Geometry: see drawing. Coordinates: mm, zero at the bounding-box minimum. A direction names the side the tool comes from. Coordinates: 2 decimals unless noted, no trailing zeros. Write each loop counter-clockwise with the first axis right and the second up, starting at its lowest first coordinate (ties: lowest second). Pieces come first, ordered by that corner, then holes. Notation, with made-up numbers: (47.5, 40.25) -> (106.5, 40.25) arc R21 ccw to (106.5, 72.25) -> close; hole circle Ø11 at (78, 37.5). An arc over 180 degrees is marked (long way). Use one line per item in the form item = value. Start each with the question number.
(1) First-contact query: pin 1 (12 mm diameter, centred on x = 38, z = 31.5, fed in from -Y); pin 2 (12.5 mm diameter, centred on y = 16.5, z = 35, fed in from +X). Flat tips, straight axial feed; report the tip coordinate or a pass-through.
(2) Ray query, line 1 along X through (y, z) = (24, 38.5); line 2 along Z through (x, y) = (36, 25); line 3 along Y through (x, z) = (43.5, 27). Return the intervals inside material, ascending.
(3) Set-up query: the marked faces 1 and 2. Return all of +Z, -Z, +X, -X, +Y, -Y with unobstructed straight access to the full face (end or side cutting, diameter ignored); none if empty.
(4) Cut plane A-A on y = 17.5. Return the cut outline in (x, z), plus the area to 3 significant figures.
(5) Cut plane B-B on x = 47. Return the cut outline in (y, z), plus the area to 3 significant figures.
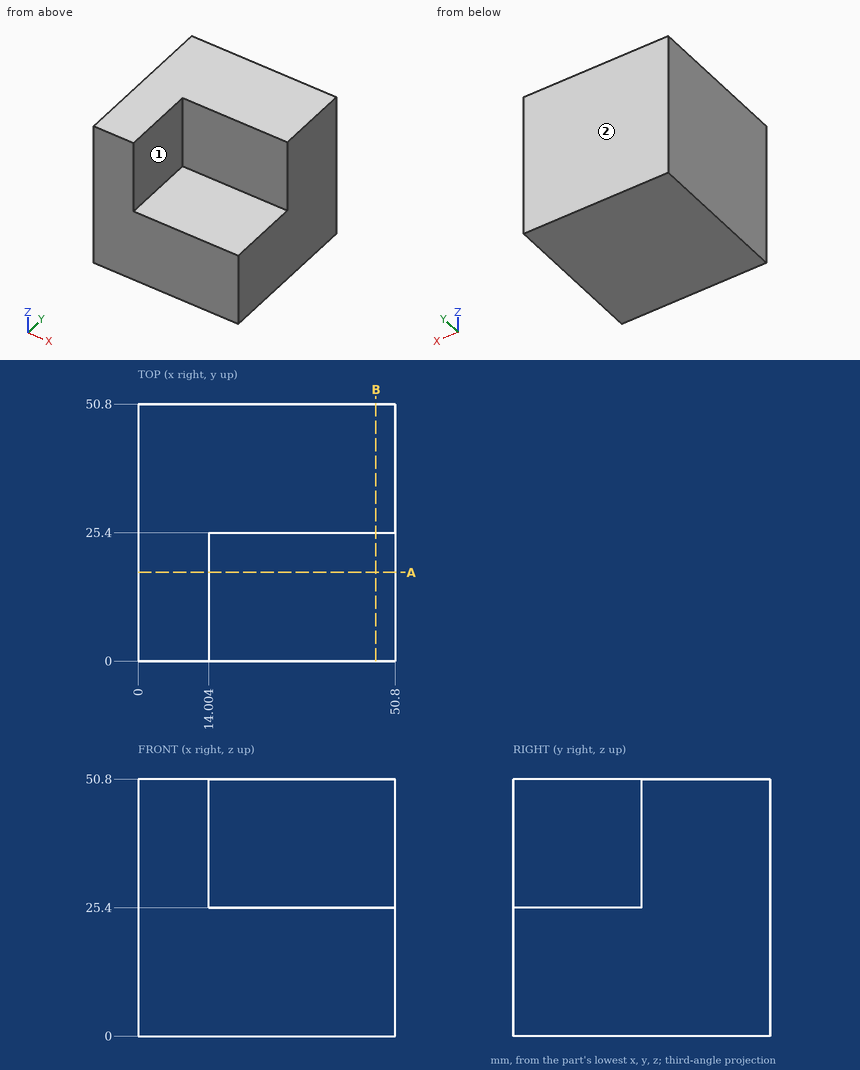
Values:
q1.pin_1 = 25.4
q1.pin_2 = 14
q2.line_1 = 0 to 14
q2.line_2 = 0 to 25.4
q2.line_3 = 25.4 to 50.8
q3.face_1 = +Z, +X, -Y
q3.face_2 = +Z, -Z, +X, -X, +Y
q4.outline = (0, 0) -> (50.8, 0) -> (50.8, 25.4) -> (14, 25.4) -> (14, 50.8) -> (0, 50.8) -> close
q4.area = 1,650 mm2
q5.outline = (0, 0) -> (50.8, 0) -> (50.8, 50.8) -> (25.4, 50.8) -> (25.4, 25.4) -> (0, 25.4) -> close
q5.area = 1,940 mm2
